Here's how the part is built. I have some questions about the finished solid (model axes, mm). A direction names the side the tool comes from. Coordinates: 2 decimals unless noted, no trailing zeros. Loops run counter-clockwise (first coordinate to the right, second up) from the corner with the lowest first, then second, coordinate; pieces in that order, holes last. Notation, with made-up numbers: (-33.5, 46) -> (-29.5, 46) arc R16 cw to (-29.5, 69) -> close; hole circle Ø1 at (65, -2). An arc over 180 degrees is marked (long way). Answer as a JSON object with one key per item and string values. Group by question number.
1) I need wall thicknesses on probe 1 along X at (y, z) = (16.5, -7.25); probe 2 along X at (y, z) = (14, -7.5); probe 3 along X at (y, z) = (11.5, -4.75). Which ranges of each line are inside material? Lowest first, please. Write a range as [from, to].
2) If we mould it in two halves opening along Z, with no side actions, what happens to faces 4 (the cylindrical face through (112.115, -1.382, -4.912)), 5 (the flat face through (95.633, 5.781, -5.028)), 6 (the flat face through (103, 17, -5)), 7 (the flat face through (107.996, 14.114, -7.465))? For each: +Z half, -Z half, draft (parallel to the pull), parting line (faces both ways), or undercut.
3) Which directions (+Z, -Z, +X, -X, +Y, -Y) give clear straight access to the entire face, cutting with the end or side of a thin tool? Please do faces 1 (the flat face through (97.663, 5.51, -1.983)), 2 (the flat face through (108.329, 17.598, -7.465)), 3 (the flat face through (76.923, 3.313, -5.028)).
4) I want a section at A-A (z = -8). Write out the boundary of the cut face in (x, y).
5) I want a section at D-D (z = -1.75). Write out the boundary of the cut face in (x, y).
6) I'm going to push flat-ended pins straight in: pin 1 (5 mm diameter, centred on y = 15.5, z = -2.5, fed in from -X); pin 2 (3 mm diameter, centred on x = 116.5, y = 16.5, fed in from +Z); pin 3 (1 mm diameter, centred on x = 108.5, z = -6.5, fed in from -Y). Where does each tip first touch, or does it pass through?
7) I want a section at C-C (y = 25.5). Write out the boundary of the cut face in (x, z), then the cut area to 3 significant figures.
8) I want a section at B-B (x = 77.5). Write out the boundary of the cut face in (y, z).
```python
from build123d import *

# Parameters (mm, degrees)
BOSS_EXTRUDE1_DEPTH = 10
SKETCH2_R           = 2
CUT_EXTRUDE1_DEPTH  = 127.229561877
CUT_EXTRUDE2_START  = -4
SKETCH2_3_R         = 2
CUT_EXTRUDE2_DEPTH  = 123.229561877
SKETCH3_R           = 2
CUT_EXTRUDE3_DEPTH  = 10
SKETCH4_R           = 2
CUT_EXTRUDE4_DEPTH  = 10
CUT_EXTRUDE5_START  = -5
SKETCH4_3_R         = 2
CUT_EXTRUDE5_DEPTH  = 5


with BuildPart() as part:
    # Sketch1 → Boss-Extrude1 (new body)
    with BuildSketch(Plane.XY):
        Polygon((125.280696375, -8.107729541), (108.169003487, 28.58841428), (53.790536264, 3.231318576), (54.697191201, 1.286990791), align=None)
    extrude(amount=-BOSS_EXTRUDE1_DEPTH)

    # Sketch2 → Cut-Extrude1 (cut, through all)
    with BuildSketch(Plane(origin=(8.369656198, -17.948785639, 0), x_dir=(0.9063077870366519, 0.4226182617406953, 0), z_dir=(-0.42261826174069533, 0.906307787036652, 0))):
        with Locations(Location((67.616396125, 5, 0), (0, 0, 180))):
            Circle(SKETCH2_R)
        with Locations(Location((92.616396125, 5, 0), (0, 0, 180))):
            Circle(SKETCH2_R)
    extrude(amount=-CUT_EXTRUDE1_DEPTH, mode=Mode.SUBTRACT)

    # Sketch2<3> → Cut-Extrude2 (cut, through all)
    # profile 1 of 2: a face of its own
    with BuildSketch(Plane(origin=(8.369656198, -17.948785639, 0), x_dir=(0.9063077870366519, 0.4226182617406953, 0), z_dir=(-0.42261826174069533, 0.906307787036652, 0)).offset(CUT_EXTRUDE2_START)):
        Polygon((92.616396125, 0.958548116), (96.116396125, 2.979274058), (96.116396125, 7.020725942), (92.616396125, 9.041451884), (89.116396125, 7.020725942), (89.116396125, 2.979274058), align=None)
        with Locations(Location((92.616396125, 5, 0), (0, 0, 180))):
            Circle(SKETCH2_3_R, mode=Mode.SUBTRACT)
    # profile 2 of 2: a face of its own
    with BuildSketch(Plane(origin=(8.369656198, -17.948785639, 0), x_dir=(0.9063077870366519, 0.4226182617406953, 0), z_dir=(-0.42261826174069533, 0.906307787036652, 0)).offset(CUT_EXTRUDE2_START)):
        Polygon((71.116396125, 2.979274058), (67.616396125, 0.958548116), (64.116396125, 2.979274058), (64.116396125, 7.020725942), (67.616396125, 9.041451884), (71.116396125, 7.020725942), align=None)
        with Locations(Location((67.616396125, 5, 0), (0, 0, 180))):
            Circle(SKETCH2_3_R, mode=Mode.SUBTRACT)
    extrude(amount=-CUT_EXTRUDE2_DEPTH, mode=Mode.SUBTRACT)

    # Sketch3 → Cut-Extrude3 (cut)
    with BuildSketch(Plane(origin=(1.120455323, 8.418096686, 0), x_dir=(0.9912580726255896, -0.1319372330110102, 0), z_dir=(-0.1319372330110102, -0.9912580726255896, 0))):
        with Locations((87.714258049, -5)):
            Circle(SKETCH3_R)
        with Locations((113.315595618, -5)):
            Circle(SKETCH3_R)
    extrude(amount=-CUT_EXTRUDE3_DEPTH, mode=Mode.SUBTRACT)

    # Sketch4 → Cut-Extrude4 (cut)
    with BuildSketch(Plane.XY):
        with Locations((105.144723808, 16.144390316)):
            Circle(SKETCH4_R)
    extrude(amount=-CUT_EXTRUDE4_DEPTH, mode=Mode.SUBTRACT)

    # Sketch4<3> → Cut-Extrude5 (cut)
    with BuildSketch(Plane.XY.offset(CUT_EXTRUDE5_START)):
        Polygon((109.170796748, 15.792154575), (107.462805377, 19.454953889), (103.436732437, 19.80718963), (101.118650868, 16.496626057), (102.826642238, 12.833826743), (106.852715178, 12.481591002), align=None)
        with Locations((105.144723808, 16.144390316)):
            Circle(SKETCH4_3_R, mode=Mode.SUBTRACT)
    extrude(amount=-CUT_EXTRUDE5_DEPTH, mode=Mode.SUBTRACT)


solid = part.part
```
Determined:
{
 "1": {"probe 1": "[82.25, 91.71], [97.92, 101.12], [108.84, 113.81]", "probe 2": "[76.88, 92.72], [98.61, 102.28], [107.92, 114.97]", "probe 3": "[71.52, 92.97], [100.69, 116.14]"},
 "2": {"face 4": "undercut", "face 5": "undercut", "face 6": "-Z half", "face 7": "draft"},
 "3": {"face 1": "none", "face 2": "-Z", "face 3": "-Y"},
 "4": {"outline": "(53.79, 3.23) -> (54.7, 1.29) -> (73.16, -1.17) -> (69.71, 6.24) -> (72.98, 7.76) -> (77.41, -1.74) -> (102.57, -5.09) -> (92.36, 16.81) -> (95.63, 18.33) -> (106.82, -5.65) -> (125.28, -8.11) -> (108.17, 28.59) -> close; hole (101.12, 16.5) -> (102.83, 12.83) -> (106.85, 12.48) -> (109.17, 15.79) -> (107.46, 19.45) -> (103.44, 19.81) -> close"},
 "5": {"outline": "(53.79, 3.23) -> (54.7, 1.29) -> (73.67, -1.24) -> (70.1, 6.42) -> (72.58, 7.58) -> (76.9, -1.67) -> (103.08, -5.15) -> (92.76, 16.99) -> (95.24, 18.15) -> (106.31, -5.58) -> (125.28, -8.11) -> (108.17, 28.59) -> close; hole circle Ø4 at (105.14, 16.14)"},
 "6": {"pin 1": "x = 74.74", "pin 2": "through", "pin 3": "y = -5.94"},
 "7": {"outline": "(101.55, -10) -> (109.61, -10) -> (109.61, 0) -> (101.55, 0) -> close", "area": "80.6 mm^2"},
 "8": {"outline": "(-1.75, -10) -> (14.29, -10) -> (14.29, 0) -> (-1.75, 0) -> (-1.75, -2.05) -> (2.08, -2.98) -> (2.08, -7.02) -> (-1.75, -7.95) -> close"}
}
